from build123d import *

# Parameters (mm, degrees)
SKETCH1_R                        = 76.2
SKETCH1_R_2                      = 6.35
SKETCH1_R_3                      = 69.85
SKETCH1_R_4                      = 20
BOSS_EXTRUDE1_DEPTH              = 69.85
SKETCH1_3_R                      = 20
CUT_EXTRUDE1_DEPTH               = 40
SKETCH1_4_R                      = 76.2
SKETCH1_4_R_2                    = 69.85
CUT_EXTRUDE2_DEPTH               = 8
SKETCH2_R                        = 40
SKETCH2_R_2                      = 30
SKETCH2_R_3                      = 27
BOSS_EXTRUDE2_DEPTH              = 32.95
SKETCH3_R                        = 32
CUT_EXTRUDE5_DEPTH               = 28
SKETCH4_R                        = 30
CUT_EXTRUDE6_DEPTH               = 22
F_1_2_14_NPSM_TAPPED_HOLE2_D     = 18.9738
F_1_2_14_NPSM_TAPPED_HOLE2_DEPTH = 41.91
CUT_EXTRUDE7_REACH               = 157.553
CUT_EXTRUDE7_END_RADIUS          = 9.4869
SKETCH12_R                       = 6.35


with BuildPart() as part:
    # Sketch1 → Boss-Extrude1 (new body)
    # profile 1 of 4: a face of its own
    with BuildSketch(Plane(origin=(0, 0, 0), x_dir=(1, 0, 0), z_dir=(0, 1, 0))):
        with BuildLine():
            ThreePointArc((79.375, 82.55), (81.62006403, 81.62006403), (82.55, 79.375))
            Line((82.55, 79.375), (82.55, -79.375))
            ThreePointArc((82.55, -79.375), (81.62006403, -81.62006403), (79.375, -82.55))
            Line((79.375, -82.55), (-79.375, -82.55))
            ThreePointArc((-79.375, -82.55), (-81.62006403, -81.62006403), (-82.55, -79.375))
            Line((-82.55, -79.375), (-82.55, 79.375))
            ThreePointArc((-82.55, 79.375), (-81.62006403, 81.62006403), (-79.375, 82.55))
            Line((-79.375, 82.55), (79.375, 82.55))
        make_face()
        Circle(SKETCH1_R, mode=Mode.SUBTRACT)
        with Locations(Location((-61.963767235, 61.963767235, 0), (0, 0, 270))):
            Circle(SKETCH1_R_2, mode=Mode.SUBTRACT)
        with Locations(Location((-61.963767235, -61.963767235, 0), (0, 0, 270))):
            Circle(SKETCH1_R_2, mode=Mode.SUBTRACT)
        with Locations(Location((61.963767235, -61.963767235, 0), (0, 0, 270))):
            Circle(SKETCH1_R_2, mode=Mode.SUBTRACT)
        with Locations(Location((61.963767235, 61.963767235, 0), (0, 0, 270))):
            Circle(SKETCH1_R_2, mode=Mode.SUBTRACT)
    # profile 2 of 4: a face of its own
    with BuildSketch(Plane(origin=(0, 0, 0), x_dir=(1, 0, 0), z_dir=(0, 1, 0))):
        Circle(SKETCH1_R)
        Circle(SKETCH1_R_3, mode=Mode.SUBTRACT)
    # profile 3 of 4: a face of its own
    with BuildSketch(Plane(origin=(0, 0, 0), x_dir=(1, 0, 0), z_dir=(0, 1, 0))):
        Circle(SKETCH1_R_3)
        Circle(SKETCH1_R_4, mode=Mode.SUBTRACT)
    # profile 4 of 4: a face of its own
    with BuildSketch(Plane(origin=(0, 0, 0), x_dir=(1, 0, 0), z_dir=(0, 1, 0))):
        Circle(SKETCH1_R_4)
    extrude(amount=BOSS_EXTRUDE1_DEPTH)

    # Sketch1<3> → Cut-Extrude1 (cut)
    with BuildSketch(Plane(origin=(0, 0, 0), x_dir=(1, 0, 0), z_dir=(0, 1, 0))):
        with Locations(Location((0, 0, 0), (0, 0, 270))):
            Circle(SKETCH1_3_R)
    extrude(amount=CUT_EXTRUDE1_DEPTH, mode=Mode.SUBTRACT)

    # Sketch1<4> → Cut-Extrude2 (cut)
    with BuildSketch(Plane(origin=(0, 0, 0), x_dir=(1, 0, 0), z_dir=(0, 1, 0))):
        with Locations(Location((0, 0, 0), (0, 0, 270))):
            Circle(SKETCH1_4_R)
        with Locations(Location((0, 0, 0), (0, 0, 270))):
            Circle(SKETCH1_4_R_2, mode=Mode.SUBTRACT)
    extrude(amount=CUT_EXTRUDE2_DEPTH, mode=Mode.SUBTRACT)

    # Sketch2 → Boss-Extrude2 (add)
    # profile 1 of 3: a face of its own
    with BuildSketch(Plane(origin=(0, 69.85, 0), x_dir=(1, 0, 0), z_dir=(0, 1, 0))):
        with Locations(Location((0, 0, 0), (0, 0, 270))):
            Circle(SKETCH2_R)
        Circle(SKETCH2_R_2, mode=Mode.SUBTRACT)
    # profile 2 of 3: a face of its own
    with BuildSketch(Plane(origin=(0, 69.85, 0), x_dir=(1, 0, 0), z_dir=(0, 1, 0))):
        Circle(SKETCH2_R_2)
        Circle(SKETCH2_R_3, mode=Mode.SUBTRACT)
    # profile 3 of 3: a face of its own
    with BuildSketch(Plane(origin=(0, 69.85, 0), x_dir=(1, 0, 0), z_dir=(0, 1, 0))):
        Circle(SKETCH2_R_3)
    extrude(amount=BOSS_EXTRUDE2_DEPTH)

    # Sketch3 → Cut-Extrude5 (cut)
    with BuildSketch(Plane(origin=(0, 102.8, 0), x_dir=(1, 0, 0), z_dir=(0, 1, 0))):
        with Locations(Location((0, 0, 0), (0, 0, 270))):
            Circle(SKETCH3_R)
    extrude(amount=-CUT_EXTRUDE5_DEPTH, mode=Mode.SUBTRACT)

    # Sketch4 → Cut-Extrude6 (cut)
    with BuildSketch(Plane(origin=(0, 74.8, 0), x_dir=(1, 0, 0), z_dir=(0, 1, 0))):
        with Locations(Location((0, 0, 0), (0, 0, 270))):
            Circle(SKETCH4_R)
    extrude(amount=-CUT_EXTRUDE6_DEPTH, mode=Mode.SUBTRACT)

    # 1/2-14 NPSM Tapped Hole2
    with Locations(Plane.ZY.offset(82.55)):
        with Locations((0, 25.4)):
            Hole(F_1_2_14_NPSM_TAPPED_HOLE2_D / 2, depth=F_1_2_14_NPSM_TAPPED_HOLE2_DEPTH)

    # Cut-Extrude7: up to this cylinder (the profile starts outside it)
    cut_extrude7_end = Plane(origin=(-50.55, 25.4, 0), z_dir=(-1, 0, 0)) * Cylinder(CUT_EXTRUDE7_END_RADIUS, 335.0798, mode=Mode.PRIVATE)
    # Sketch12 → Cut-Extrude7 (cut, up to the surface)
    with BuildSketch(Plane.XZ, mode=Mode.PRIVATE) as cut_extrude7_sk1:
        with Locations(Location((-50.55, 0, 0), (0, 0, 270))):
            Circle(SKETCH12_R)
    cut_extrude7_tool1 = extrude(cut_extrude7_sk1.sketch, amount=-CUT_EXTRUDE7_REACH, mode=Mode.PRIVATE) - cut_extrude7_end
    add(cut_extrude7_tool1.solids().sort_by_distance((-50.55, 0, 0))[0], mode=Mode.SUBTRACT)


solid = part.part
The model under review builds one solid part; all positions refer to its coordinate system, in mm. A direction names the side the tool comes from. Round coordinates to 2 decimals unless told otherwise and drop trailing zeros. Loops run counter-clockwise (first coordinate to the right, second up) from the corner with the lowest first, then second, coordinate; pieces in that order, holes last. Notation, with made-up numbers: (21.5, 11) -> (34.5, 11) arc R9 ccw to (34.5, 23) -> close; hole circle Ø2 at (-29.75, 16.25). An arc over 180 degrees is marked (long way). Return JSON: item names as keys, results as strings.
(1) For line 1 (X direction, y = 2.75, z = 0); line 2 (X direction, y = 27.5, z = 0); line 3 (Z direction, x = -50.55, y = 11.5), list the stretches that pass through material, from the lowest coordinate up.
Solved:
{"line 1": "-82.55 to -76.2, -69.85 to -56.9, -44.2 to -20, 20 to 69.85, 76.2 to 82.55", "line 2": "-40.64 to -20, 20 to 82.55", "line 3": "-82.55 to -6.35, 6.35 to 82.55"}
(2) Add section C-C on z = -23. Write out the cut boundary in (x, y), plus the area to 3 significant figures.
Solved:
{"outline": "(-82.55, 0) -> (-72.65, 0) -> (-72.65, 8) -> (-65.95, 8) -> (-65.95, 0) -> (65.95, 0) -> (65.95, 8) -> (72.65, 8) -> (72.65, 0) -> (82.55, 0) -> (82.55, 69.85) -> (32.73, 69.85) -> (32.73, 102.8) -> (22.25, 102.8) -> (22.25, 74.8) -> (19.26, 74.8) -> (19.26, 52.8) -> (-19.26, 52.8) -> (-19.26, 74.8) -> (-22.25, 74.8) -> (-22.25, 102.8) -> (-32.73, 102.8) -> (-32.73, 69.85) -> (-82.55, 69.85) -> close", "area": "11,500 mm2"}
(3) For pin 1 (10 mm diameter, centred on x = -50.55, z = 0, fed in from +Y); pin 2 (10 mm diameter, centred on x = 61.96, z = 61.96, fed in from -Y), all flat-tipped, find the tip position at first contact; note any pin that passes through.
Solved:
{"pin 1": "y = 69.85", "pin 2": "through"}
(4) Add section A-A on x = 0. Write out the cut boundary in (y, z), plus the area to 3 significant figures.
Solved:
{"outline": "(0, -82.55) -> (69.85, -82.55) -> (69.85, -40) -> (102.8, -40) -> (102.8, -32) -> (74.8, -32) -> (74.8, -30) -> (52.8, -30) -> (52.8, 30) -> (74.8, 30) -> (74.8, 32) -> (102.8, 32) -> (102.8, 40) -> (69.85, 40) -> (69.85, 82.55) -> (0, 82.55) -> (0, 76.2) -> (8, 76.2) -> (8, 69.85) -> (0, 69.85) -> (0, 20) -> (40, 20) -> (40, -20) -> (0, -20) -> (0, -69.85) -> (8, -69.85) -> (8, -76.2) -> (0, -76.2) -> close", "area": "9,350 mm2"}
(5) Add section B-B on y = 25.4. Write out the cut boundary in (x, z) (3 decimals), plus the area to 3 significant figures.
Solved:
{"outline": "(-82.55, -79.375) arc R3.175 ccw to (-79.375, -82.55) -> (79.375, -82.55) arc R3.175 ccw to (82.55, -79.375) -> (82.55, 79.375) arc R3.175 ccw to (79.375, 82.55) -> (-79.375, 82.55) arc R3.175 ccw to (-82.55, 79.375) -> (-82.55, 9.487) -> (-40.64, 9.487) -> (-40.64, -9.487) -> (-82.55, -9.487) -> close; hole circle Ø12.7 at (-61.964, -61.964); hole circle Ø12.7 at (-61.964, 61.964); hole circle Ø40 at (0, 0); hole circle Ø12.7 at (61.964, -61.964); hole circle Ø12.7 at (61.964, 61.964)", "area": "24,700 mm2"}
(6) The part is to be moulded in two halves that separate along Z. For faces 1 (the flat face through (-62, 8, 34)), 2 (the flat face through (38, 69.85, -20)), 3 (the flat face through (1, 34, 82.55)), say which applies: released by +Z, released by -Z, zero draft, split by the parting line, or undercut.
Solved:
{"face 1": "undercut", "face 2": "zero draft", "face 3": "released by +Z"}
(7) Add section D-D on x = -50.55. Write out the cut boundary in (y, z), plus the area to 3 significant figures.
Solved:
{"outline": "(0, -82.55) -> (69.85, -82.55) -> (69.85, 82.55) -> (0, 82.55) -> (0, 57.02) -> (8, 57.02) -> (8, 48.2) -> (0, 48.2) -> (0, 6.35) -> (18.35, 6.35) arc R9.49 cw (long way) to (18.35, -6.35) -> (0, -6.35) -> (0, -48.2) -> (8, -48.2) -> (8, -57.02) -> (0, -57.02) -> close", "area": "10,900 mm2"}
(8) For faces 4 (the cylindrical face through (-19.524, 19.72, -4.336)), 5 (the flat face through (-40.64, 26, 0)), 6 (the flat face through (0, 52.8, 0)), 7 (the flat face through (15, 0, 15)), list the 3-axis set-ups (+Z, -Z, +X, -X, +Y, -Y) from which the entire face can be reached by the end or side of a thin tool; tool diameter is ignored.
Solved:
{"face 4": "-Y", "face 5": "-X", "face 6": "+Y", "face 7": "+Z, -Z, +X, -X, -Y"}
